Here's how the part is built. I have some questions about the finished solid (model axes, mm). Round coordinates to 2 decimals unless told otherwise and drop trailing zeros. Use one line per item in the form item = value. Start each with the question number.
Item 1: If I drill on L1, parallel to Z at x = -144.75, y = 1.7, over which ranges is the centre line in solid material (lowest first)? Write a range as [from, to].
Item 2: If we section it at A-A (z = 16): State how many separate pieces and enclosed holes the cut face has, then the cut area to 3 significant figures.
Item 3: I'm going to push a flat-ended pin straight in: pin 1 Ø0.5 at (x, y) = (-139, 2.5) entering from +Z. Where does the tip first touch, or does it pass through?
```python
from build123d import *

# Parameters (mm, degrees)
SKETCH3_R           = 1.4
BOSS_EXTRUDE1_DEPTH = 3.175


with BuildPart() as part:
    # Sketch3 → Boss-Extrude1 (new body)
    with BuildSketch(Plane(origin=(0, 0, 0), x_dir=(1, 0, 0), z_dir=(0, 1, 0))):
        with BuildLine():
            Line((-72.55, 42), (-71.45, 42))
            Line((-71.45, 42), (-71.45, -50))
            Line((-71.45, -50), (-62.95, -50))
            Line((-62.95, -50), (-62.95, 42))
            Line((-62.95, 42), (-61.85, 42))
            Line((-61.85, 42), (-61.85, -50))
            Line((-61.85, -50), (-53.35, -50))
            Line((-53.35, -50), (-53.35, 42))
            Line((-53.35, 42), (-52.25, 42))
            Line((-52.25, 42), (-52.25, -50))
            Line((-52.25, -50), (-43.75, -50))
            Line((-43.75, -50), (-43.75, 42))
            Line((-43.75, 42), (-42.65, 42))
            Line((-42.65, 42), (-42.65, -50))
            Line((-42.65, -50), (-34.15, -50))
            Line((-34.15, -50), (-34.15, 42))
            Line((-34.15, 42), (-33.05, 42))
            Line((-33.05, 42), (-33.05, -50))
            Line((-33.05, -50), (-24.55, -50))
            Line((-24.55, -50), (-24.55, 42))
            Line((-24.55, 42), (-23.45, 42))
            Line((-23.45, 42), (-23.45, -50))
            Line((-23.45, -50), (-14.95, -50))
            Line((-14.95, -50), (-14.95, 42))
            Line((-14.95, 42), (-13.85, 42))
            Line((-13.85, 42), (-13.85, -50))
            Line((-13.85, -50), (-5.35, -50))
            Line((-5.35, -50), (-5.35, 42))
            Line((-5.35, 42), (-4.25, 42))
            Line((-4.25, 42), (-4.25, -50))
            Line((-4.25, -50), (4.25, -50))
            Line((4.25, -50), (4.25, 42))
            Line((4.25, 42), (5.35, 42))
            Line((5.35, 42), (5.35, -50))
            Line((5.35, -50), (13.85, -50))
            Line((13.85, -50), (13.85, 42))
            Line((13.85, 42), (14.95, 42))
            Line((14.95, 42), (14.95, -50))
            Line((14.95, -50), (23.45, -50))
            Line((23.45, -50), (23.45, 42))
            Line((23.45, 42), (24.55, 42))
            Line((24.55, 42), (24.55, -50))
            Line((24.55, -50), (33.05, -50))
            Line((33.05, -50), (33.05, 42))
            Line((33.05, 42), (34.15, 42))
            Line((34.15, 42), (34.15, -50))
            Line((34.15, -50), (42.65, -50))
            Line((42.65, -50), (42.65, 42))
            Line((42.65, 42), (43.75, 42))
            Line((43.75, 42), (43.75, -50))
            Line((43.75, -50), (52.25, -50))
            Line((52.25, -50), (52.25, 42))
            Line((52.25, 42), (53.35, 42))
            Line((53.35, 42), (53.35, -50))
            Line((53.35, -50), (61.85, -50))
            Line((61.85, -50), (61.85, 42))
            Line((61.85, 42), (62.95, 42))
            Line((62.95, 42), (62.95, -50))
            Line((62.95, -50), (71.45, -50))
            Line((71.45, -50), (71.45, 42))
            Line((71.45, 42), (72.55, 42))
            Line((72.55, 42), (72.55, -50))
            Line((72.55, -50), (81.05, -50))
            Line((81.05, -50), (81.05, 42))
            Line((81.05, 42), (82.15, 42))
            Line((82.15, 42), (82.15, -50))
            Line((82.15, -50), (90.65, -50))
            Line((90.65, -50), (90.65, 42))
            Line((90.65, 42), (91.75, 42))
            Line((91.75, 42), (91.75, -50))
            Line((91.75, -50), (100.25, -50))
            Line((100.25, -50), (100.25, 42))
            Line((100.25, 42), (101.35, 42))
            Line((101.35, 42), (101.35, -50))
            Line((101.35, -50), (109.85, -50))
            Line((109.85, -50), (109.85, 42))
            Line((109.85, 42), (110.95, 42))
            Line((110.95, 42), (110.95, -50))
            Line((110.95, -50), (119.45, -50))
            Line((119.45, -50), (119.45, 42))
            Line((119.45, 42), (120.55, 42))
            Line((120.55, 42), (120.55, -50))
            Line((120.55, -50), (129.05, -50))
            Line((129.05, -50), (129.05, 42))
            Line((129.05, 42), (130.15, 42))
            Line((130.15, 42), (130.15, -50))
            Line((130.15, -50), (138.65, -50))
            Line((138.65, -50), (138.65, 42))
            Line((138.65, 42), (139.75, 42))
            Line((139.75, 42), (139.75, -50))
            Line((139.75, -50), (147.25, -50))
            ThreePointArc((147.25, -50), (149.017766953, -49.267766953), (149.75, -47.5))
            Line((149.75, -47.5), (149.75, 47.5))
            ThreePointArc((149.75, 47.5), (149.017766953, 49.267766953), (147.25, 50))
            Line((147.25, 50), (-147.25, 50))
            ThreePointArc((-147.25, 50), (-149.017766953, 49.267766953), (-149.75, 47.5))
            Line((-149.75, 47.5), (-149.75, -47.5))
            ThreePointArc((-149.75, -47.5), (-149.017766953, -49.267766953), (-147.25, -50))
            Line((-147.25, -50), (-139.75, -50))
            Line((-139.75, -50), (-139.75, 42))
            Line((-139.75, 42), (-138.65, 42))
            Line((-138.65, 42), (-138.65, -50))
            Line((-138.65, -50), (-130.15, -50))
            Line((-130.15, -50), (-130.15, 42))
            Line((-130.15, 42), (-129.05, 42))
            Line((-129.05, 42), (-129.05, -50))
            Line((-129.05, -50), (-120.55, -50))
            Line((-120.55, -50), (-120.55, 42))
            Line((-120.55, 42), (-119.45, 42))
            Line((-119.45, 42), (-119.45, -50))
            Line((-119.45, -50), (-110.95, -50))
            Line((-110.95, -50), (-110.95, 42))
            Line((-110.95, 42), (-109.85, 42))
            Line((-109.85, 42), (-109.85, -50))
            Line((-109.85, -50), (-101.35, -50))
            Line((-101.35, -50), (-101.35, 42))
            Line((-101.35, 42), (-100.25, 42))
            Line((-100.25, 42), (-100.25, -50))
            Line((-100.25, -50), (-91.75, -50))
            Line((-91.75, -50), (-91.75, 42))
            Line((-91.75, 42), (-90.65, 42))
            Line((-90.65, 42), (-90.65, -50))
            Line((-90.65, -50), (-82.15, -50))
            Line((-82.15, -50), (-82.15, 42))
            Line((-82.15, 42), (-81.05, 42))
            Line((-81.05, 42), (-81.05, -50))
            Line((-81.05, -50), (-72.55, -50))
            Line((-72.55, -50), (-72.55, 42))
        make_face()
        with Locations(Location((-144.75, -40, 0), (0, 0, 270))):
            Circle(SKETCH3_R, mode=Mode.SUBTRACT)
        with Locations(Location((-48, -40, 0), (0, 0, 270))):
            Circle(SKETCH3_R, mode=Mode.SUBTRACT)
        with Locations(Location((48, -40, 0), (0, 0, 270))):
            Circle(SKETCH3_R, mode=Mode.SUBTRACT)
        with Locations(Location((144.75, -40, 0), (0, 0, 270))):
            Circle(SKETCH3_R, mode=Mode.SUBTRACT)
        with Locations(Location((-144.75, 40, 0), (0, 0, 270))):
            Circle(SKETCH3_R, mode=Mode.SUBTRACT)
        with Locations(Location((0, 40, 0), (0, 0, 270))):
            Circle(SKETCH3_R, mode=Mode.SUBTRACT)
        with Locations(Location((144.75, 40, 0), (0, 0, 270))):
            Circle(SKETCH3_R, mode=Mode.SUBTRACT)
    extrude(amount=BOSS_EXTRUDE1_DEPTH)


solid = part.part
```
Values found:
q1.L1 = [-50, -41.4], [-38.6, 38.6], [41.4, 50]
q2.separate_pieces = 31
q2.enclosed_holes = 0
q2.area = 846 mm2
q3.pin_1 = -42
